Answer from the drawing. Dimensions are ordinates in mm from the lowest x, y and z of the part. A direction names the side the tool comes from. Round coordinates to 2 decimals unless told otherwise and drop trailing zeros. Loops run counter-clockwise (first coordinate to the right, second up) from the corner with the lowest first, then second, coordinate; pieces in that order, holes last.
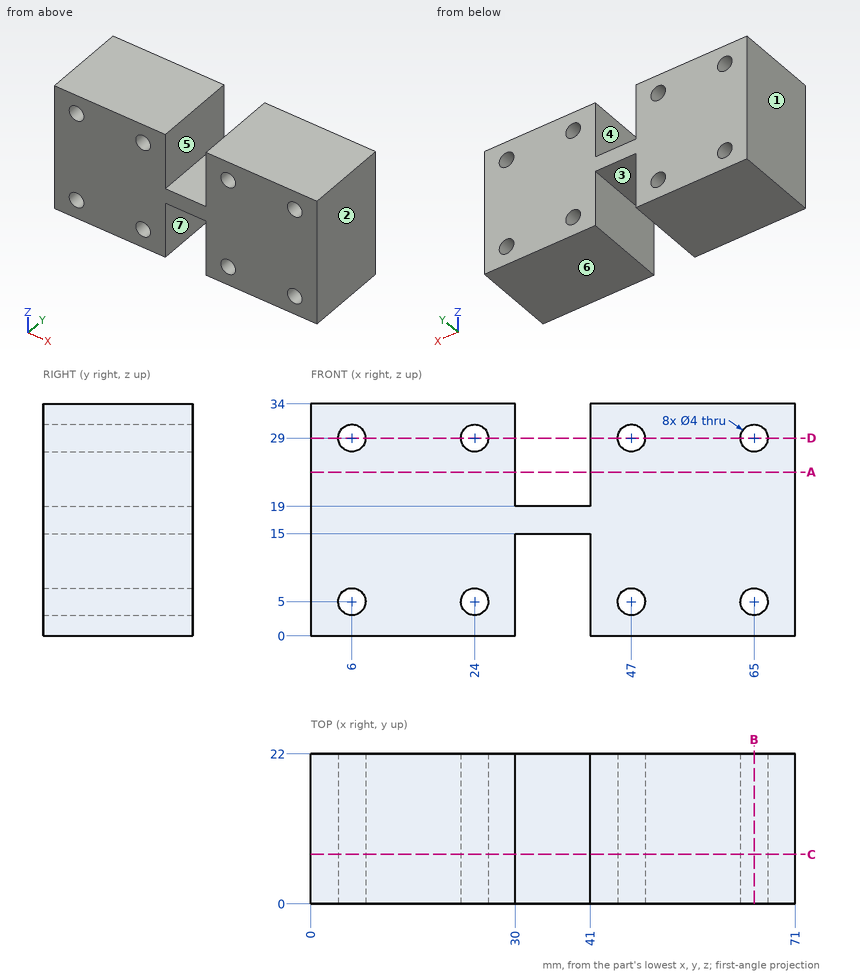
1. Given pin 1 (3 mm diameter, centred on y = 12, z = 29, fed in from -X); pin 2 (9 mm diameter, centred on x = 35.5, y = 11, fed in from +Z), each flat-ended and moving along its own axis, determine where each tip first touches the part or whether it passes through.
Answer key:
pin 1: stops at x = 0
pin 2: stops at z = 19
2. Consider probe 1 along X at (y, z) = (7, 5); probe 2 along X at (y, z) = (14.75, 9); probe 3 along Z at (x, y) = (23.5, 8.75). Determine where each line is inside the solid, lowest interval first.
Answer key:
probe 1: x = 0 to 4, 8 to 22, 26 to 30, 41 to 45, 49 to 63, 67 to 71
probe 2: x = 0 to 30, 41 to 71
probe 3: z = 0 to 3.06, 6.94 to 27.06, 30.94 to 34
3. Find section B-B (x = 65). Write down the section's boundary in (y, z).
Answer key:
outline: (0, 0) - (22, 0) - (22, 3) - (0, 3) - close; (0, 7) - (22, 7) - (22, 27) - (0, 27) - close; (0, 31) - (22, 31) - (22, 34) - (0, 34) - close
4. Find section C-C (y = 7.25). Give the number of separate pieces and of enclosed holes in the cut face, then the cut area to 3 significant figures.
Answer key:
separate pieces: 1
enclosed holes: 8
area: 1,980 mm2
5. Find section A-A (z = 24). Write down the section's boundary in (x, y).
Answer key:
outline: (0, 0) - (30, 0) - (30, 22) - (0, 22) - close; (41, 0) - (71, 0) - (71, 22) - (41, 22) - close
6. Find section D-D (z = 29). Write down the section's boundary in (x, y).
Answer key:
outline: (0, 0) - (4, 0) - (4, 22) - (0, 22) - close; (8, 0) - (22, 0) - (22, 22) - (8, 22) - close; (26, 0) - (30, 0) - (30, 22) - (26, 22) - close; (41, 0) - (45, 0) - (45, 22) - (41, 22) - close; (49, 0) - (63, 0) - (63, 22) - (49, 22) - close; (67, 0) - (71, 0) - (71, 22) - (67, 22) - close
7. Determine the mould class of the marked faces 1, 2, 3 and 4 for opening direction X: +X half, -X half, draft (parallel to the pull), parting line (faces both ways), or undercut.
Answer key:
face 1: -X half
face 2: +X half
face 3: undercut
face 4: undercut
8. Which of the six approach directions +Z, -Z, +X, -X, +Y, -Y give full straight-line access (tool end or side, diameter ignored) to the marked faces 5, 6 and 7?
Answer key:
face 5: +Z, +Y, -Y
face 6: -Z, +X, -X, +Y, -Y
face 7: -Z, +Y, -Y
